CAD build for the part. Positions are in the model's coordinates, mm. Face numbers are marked on the shaded views. A direction names the side the tool comes from. Give positions to 0.01 mm unless a question says otherwise; leave off trailing zeros. Loops run counter-clockwise (first coordinate to the right, second up) from the corner with the lowest first, then second, coordinate; pieces in that order, holes last. Notation, with made-up numbers: (36.5, 57) -> (81.5, 57) arc R34 ccw to (81.5, 89) -> close; hole circle Ø10 at (42, -10.5). An arc over 180 degrees is marked (long way). Use one line per item in the form item = value.
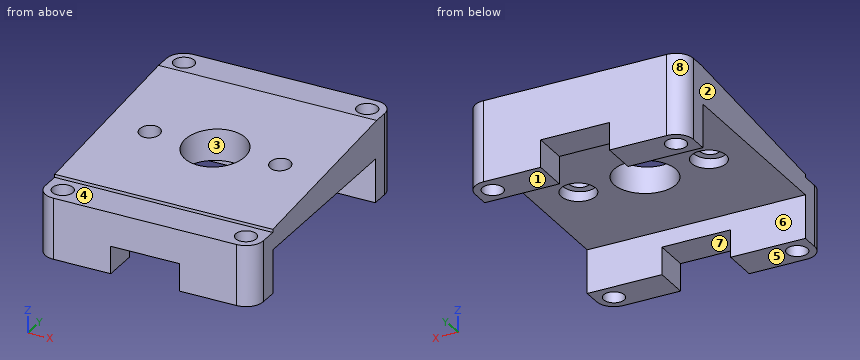
```python
from build123d import *

# Parameters (mm, degrees)
F0_R      = 1.5
F0_R_2    = 4.5
F1_DEPTH  = 2.54
F2_R      = 1.5
F3_DEPTH  = 6.35
F4_W      = 10
F4_H      = 4
F5_DEPTH  = 38.101
F7_DEPTH  = 25.4
F8_W      = 55.4393846542
F8_H      = 54.9912601709
F9_DEPTH  = 25.4
F10_R     = 1.5
F11_DEPTH = 25.4
F13_R     = 2.5
F13_R_2   = 1.5
F14_DEPTH = 25.4
F16_W     = 46.2689362466
F16_H     = 11.2376865
F17_DEPTH = 25.4
F19_W     = 33.8024366647
F19_H     = 5.08
F20_DEPTH = 25.4


with BuildPart() as f1:
    # F0 (on Top) → F1 (new body)
    with BuildSketch(Plane.XY):
        with BuildLine():
            ThreePointArc((15.875, 16.51), (15.1310512242, 18.3060512242), (13.335, 19.05))
            Line((13.335, 19.05), (-13.335, 19.05))
            ThreePointArc((-13.335, 19.05), (-15.1310512242, 18.3060512242), (-15.875, 16.51))
            Line((-15.875, 16.51), (-15.875, -16.51))
            ThreePointArc((-15.875, -16.51), (-15.1310512242, -18.3060512242), (-13.335, -19.05))
            Line((-13.335, -19.05), (13.335, -19.05))
            ThreePointArc((13.335, -19.05), (15.1310512242, -18.3060512242), (15.875, -16.51))
            Line((15.875, -16.51), (15.875, 16.51))
        make_face()
        with Locations((-13.335, -16.51)):
            Circle(F0_R, mode=Mode.SUBTRACT)
        with Locations((13.335, -16.51)):
            Circle(F0_R, mode=Mode.SUBTRACT)
        with Locations((-13.335, 16.51)):
            Circle(F0_R, mode=Mode.SUBTRACT)
        Circle(F0_R_2, mode=Mode.SUBTRACT)
        with Locations((13.335, 16.51)):
            Circle(F0_R, mode=Mode.SUBTRACT)
    extrude(amount=F1_DEPTH)

    # F2 (on face) → F3 (join)
    with BuildSketch(Plane(origin=(0, 0, 0), x_dir=(1, 0, 0), z_dir=(0, 0, -1))):
        with BuildLine():
            Line((-15.875, 16.51), (-15.875, 13.97))
            Line((-15.875, 13.97), (15.875, 13.97))
            Line((15.875, 13.97), (15.875, 16.51))
            ThreePointArc((15.875, 16.51), (15.1310512242, 18.3060512242), (13.335, 19.05))
            Line((13.335, 19.05), (-13.335, 19.05))
            ThreePointArc((-13.335, 19.05), (-15.1310512242, 18.3060512242), (-15.875, 16.51))
        make_face()
        with Locations((-13.335, 16.51)):
            Circle(F2_R, mode=Mode.SUBTRACT)
        with Locations((13.335, 16.51)):
            Circle(F2_R, mode=Mode.SUBTRACT)
        with BuildLine():
            Line((15.875, -13.97), (-15.875, -13.97))
            Line((-15.875, -13.97), (-15.875, -16.51))
            ThreePointArc((-15.875, -16.51), (-15.1310512242, -18.3060512242), (-13.335, -19.05))
            Line((-13.335, -19.05), (13.335, -19.05))
            ThreePointArc((13.335, -19.05), (15.1310512242, -18.3060512242), (15.875, -16.51))
            Line((15.875, -16.51), (15.875, -13.97))
        make_face()
        with Locations((-13.335, -16.51)):
            Circle(F2_R, mode=Mode.SUBTRACT)
        with Locations((13.335, -16.51)):
            Circle(F2_R, mode=Mode.SUBTRACT)
    extrude(amount=F3_DEPTH)

    # F4 (on face) → F5 (cut, through all)
    with BuildSketch(Plane(origin=(0, 19.05, 0), x_dir=(-1, 0, 0), z_dir=(0, 1, 0))):
        with Locations((0, -4.35)):
            Rectangle(F4_W, F4_H)
    extrude(amount=-F5_DEPTH, mode=Mode.SUBTRACT)

    # F7 (add): a face of the model
    f7_faces = [f1.faces().sort_by_distance(p)[0] for p in [
        (14.7803610119, 17.9553610119, 2.54),
    ]]
    extrude(f7_faces, amount=F7_DEPTH)

    # F8 (on face) → F9 (cut)
    with BuildSketch(Plane(origin=(0, -0.3652393382, 4.1747047386), x_dir=(1, 0, 0), z_dir=(0, -0.0871557427, 0.9961946981))):
        with Locations((6.7749572918, -4.9830414355)):
            Rectangle(F8_W, F8_H)
    extrude(amount=F9_DEPTH, mode=Mode.SUBTRACT)

    # F10 (on face) → F11 (cut)
    with BuildSketch(Plane(origin=(0, -0.3652393382, 4.1747047386), x_dir=(1, 0, 0), z_dir=(0, -0.0871557427, 0.9961946981))):
        with Locations((-9.5, 0.3666344931)):
            Circle(F10_R)
        with BuildLine():
            ThreePointArc((11, 0.3666344931), (9.5, 1.8666344931), (8, 0.3666344931))
            ThreePointArc((8, 0.3666344931), (9.5, -1.1333655069), (11, 0.3666344931))
        make_face()
    extrude(amount=-F11_DEPTH, mode=Mode.SUBTRACT)

    # F13 (on offset) → F14 (cut)
    with BuildSketch(Plane(origin=(0, -0.1438637516, 1.6443702054), x_dir=(1, 0, 0), z_dir=(0, -0.0871557427, 0.9961946981))):
        with Locations((-9.5, 0.3666344931)):
            Circle(F13_R)
        with Locations((-9.5, 0.3666344931)):
            Circle(F13_R_2, mode=Mode.SUBTRACT)
        with Locations((9.5, 0.3666344931)):
            Circle(F13_R)
        with Locations((9.5, 0.3666344931)):
            Circle(F13_R_2, mode=Mode.SUBTRACT)
    extrude(amount=-F14_DEPTH, mode=Mode.SUBTRACT)

    # F16 (on offset) → F17 (cut)
    with BuildSketch(Plane(origin=(0, 0, 5.461), x_dir=(1, 0, 0), z_dir=(0, 0, -1))):
        with Locations((-5.8952979743, -18.3988427743)):
            Rectangle(F16_W, F16_H)
    extrude(amount=-F17_DEPTH, mode=Mode.SUBTRACT)

    # F19 (on offset) → F20 (cut)
    with BuildSketch(Plane(origin=(0, 0, 2.54), x_dir=(1, 0, 0), z_dir=(0, 0, -1))):
        with Locations((1.0262183324, 16.51)):
            Rectangle(F19_W, F19_H)
    extrude(amount=-F20_DEPTH, mode=Mode.SUBTRACT)


solid = f1.part
```
1. Mould opens along X. For the marked faces 1, 2 and 3 say: pulls with the +X half, pulls with the -X half, needs draft (parallel to the pull), parting line crosses it, or undercut.
Result sheet:
face_1 = needs draft
face_2 = pulls with the -X half
face_3 = undercut
2. Cut at A-A, the plane z = -3. Write the cut outline in (x, y) (3 decimals).
Result sheet:
outline = (-15.875, -16.51) arc R2.54 ccw to (-13.335, -19.05) -> (-5, -19.05) -> (-5, -13.97) -> (-15.875, -13.97) -> close; (-15.875, 13.97) -> (-5, 13.97) -> (-5, 19.05) -> (-13.335, 19.05) arc R2.54 ccw to (-15.875, 16.51) -> close; (5, -19.05) -> (13.335, -19.05) arc R2.54 ccw to (15.875, -16.51) -> (15.875, -13.97) -> (5, -13.97) -> close; (5, 13.97) -> (15.875, 13.97) -> (15.875, 16.51) arc R2.54 ccw to (13.335, 19.05) -> (5, 19.05) -> close; hole circle Ø3 at (-13.335, -16.51); hole circle Ø3 at (-13.335, 16.51); hole circle Ø3 at (13.335, -16.51); hole circle Ø3 at (13.335, 16.51)
3. Cut at C-C, the plane x = 1. Write the cut outline in (y, z).
Result sheet:
outline = (-19.05, -2.35) -> (-13.97, -2.35) -> (-13.97, 0) -> (-4.39, 0) -> (-4.39, 3.82) -> (-13.97, 2.98) -> (-13.97, 2.54) -> (-19.05, 2.54) -> close; (4.39, 0) -> (13.97, 0) -> (13.97, -2.35) -> (19.05, -2.35) -> (19.05, 5.46) -> (14.34, 5.46) -> (4.39, 4.59) -> close
4. Cut at D-D, the plane y = 4. Write the cut outline in (x, z) (3 decimals), then the cut area to 3 significant figures.
Result sheet:
outline = (-15.875, 0) -> (-2.062, 0) -> (-2.062, 4.557) -> (-15.875, 4.557) -> close; (2.062, 0) -> (15.875, 0) -> (15.875, 4.557) -> (2.062, 4.557) -> close
area = 126 mm^2
5. Drop flat-ended pins along their axis: P1, Ø4, axis at x = -2.5, y = -17.5, coming from the +Z side; P2, Ø5.5, axis at x = 0.5, y = 16, coming from the -Z side; P3, Ø4.5, axis at y = -17.5, z = -5, coming from the +X side (3 decimals); P4, Ø8.5, axis at x = -2.5, y = -2.5, coming from the -Z side. Give the stop position or say it passes through.
Result sheet:
P1 = 2.54
P2 = -2.35
P3 = 15.875
P4 = 0
6. Tool access for the marked faces 4, 5, 6, 7 and 8: list every direction of +Z, -Z, +X, -X, +Y, -Y with a clear straight run to the whole face (end or side of a thin tool).
Result sheet:
face_4 = +Z, +X, -X, -Y
face_5 = -Z, +X, -X, +Y, -Y
face_6 = -Z, +X, -X
face_7 = -Z, +Y, -Y
face_8 = +Z, -Z, -X, +Y
7. Drill centre lines: line 1 (X direction, y = 0, z = 3.3) (3 decimals); line 2 (X direction, y = -16.51, z = -3.5) (3 decimals); line 3 (X direction, y = -16.51, z = 0.5) (3 decimals). Where is each one in solid material? Low to high.
Result sheet:
line_1 = -15.875 to -10.998, -8.002 to -4.5, 4.5 to 8.002, 10.998 to 15.875
line_2 = -15.875 to -14.835, -11.835 to -5, 5 to 11.835, 14.835 to 15.875
line_3 = -15.875 to -14.835, -11.835 to 11.835, 14.835 to 15.875
8. Cut at B-B, the plane x = 14. Write the cut outline in (y, z), then the cut area to 3 significant figures.
Result sheet:
outline = (-18.96, -6.35) -> (-17.85, -6.35) -> (-17.85, 2.54) -> (-18.96, 2.54) -> close; (-15.17, -6.35) -> (-13.97, -6.35) -> (-13.97, 0) -> (13.97, 0) -> (13.97, -6.35) -> (15.17, -6.35) -> (15.17, 5.46) -> (14.34, 5.46) -> (-13.97, 2.98) -> (-13.97, 2.54) -> (-15.17, 2.54) -> close; (17.85, -6.35) -> (18.96, -6.35) -> (18.96, 5.46) -> (17.85, 5.46) -> close
area = 165 mm^2
